from build123d import *

# Parameters (mm, degrees)
BOSS_EXTRUDE1_DEPTH = 3
SKETCH2_R           = 1.5
SKETCH2_W           = 57.5
SKETCH2_H           = 86
CUT_EXTRUDE1_DEPTH  = 102.651364969
SKETCH3_W           = 3
SKETCH3_H           = 15
CUT_EXTRUDE2_DEPTH  = 102.651364969


with BuildPart() as part:
    # Sketch1 → Boss-Extrude1 (new body)
    with BuildSketch(Plane(origin=(0, 0, 0), x_dir=(1, 0, 0), z_dir=(0, 1, 0))):
        with BuildLine():
            Line((-74, 60), (74, 60))
            ThreePointArc((74, 60), (79.656854249, 57.656854249), (82, 52))
            Line((82, 52), (82, -52))
            ThreePointArc((82, -52), (79.656854249, -57.656854249), (74, -60))
            Line((74, -60), (-74, -60))
            ThreePointArc((-74, -60), (-79.656854249, -57.656854249), (-82, -52))
            Line((-82, -52), (-82, 52))
            ThreePointArc((-82, 52), (-79.656854249, 57.656854249), (-74, 60))
        make_face()
    extrude(amount=BOSS_EXTRUDE1_DEPTH)

    # Sketch2 → Cut-Extrude1 (cut, through all)
    with BuildSketch(Plane(origin=(0, 3, 0), x_dir=(1, 0, 0), z_dir=(0, 1, 0))):
        with Locations(Location((-38.25, 50, 0), (0, 0, 270))):
            Circle(SKETCH2_R)
        with Locations(Location((-38.25, -50, 0), (0, 0, 270))):
            Circle(SKETCH2_R)
        with Locations((-38.25, -1.5)):
            Rectangle(SKETCH2_W, SKETCH2_H)
    extrude(amount=-CUT_EXTRUDE1_DEPTH, mode=Mode.SUBTRACT)

    # Sketch3 → Cut-Extrude2 (cut, through all)
    with BuildSketch(Plane(origin=(0, 3, 0), x_dir=(1, 0, 0), z_dir=(0, 1, 0))):
        with Locations((-72.5, 32.5)):
            Rectangle(SKETCH3_W, SKETCH3_H)
        with Locations((-72.5, -32.5)):
            Rectangle(SKETCH3_W, SKETCH3_H)
        with Locations((72.5, -32.5)):
            Rectangle(SKETCH3_W, SKETCH3_H)
        with Locations((72.5, 32.5)):
            Rectangle(SKETCH3_W, SKETCH3_H)
    extrude(amount=-CUT_EXTRUDE2_DEPTH, mode=Mode.SUBTRACT)


solid = part.part
Verification items for the finished model (mm, model axes). Round coordinates to 2 decimals unless told otherwise and drop trailing zeros. Loops run counter-clockwise (first coordinate to the right, second up) from the corner with the lowest first, then second, coordinate; pieces in that order, holes last. Notation, with made-up numbers: (-15.5, 56.5) - (34.5, 56.5) arc R26 ccw to (34.5, 81.5) - close; hole circle Ø1 at (65, -7). An arc over 180 degrees is marked (long way). Use a Markdown table: item, result. Add a question column.
1. Section check B-B, the plane z = -31. Record the boundary of the cut face in (x, y), plus the area to 4 significant figures.
2. Thickness scan on probe 1 along X at (y, z) = (0.6, 30.5); probe 2 along X at (y, z) = (1.35, 4); probe 3 along Z at (x, y) = (-13, 1.1). Record the ranges inside material, lowest first. Write a range as [from, to].
3. Gauge pin test, flat end, axial feed: pin 1 (2.5 mm diameter, centred on x = -38.25, z = -50, fed in from +Y). Record the tip position at first contact, or that the pin passes through.
4. Section check A-A, the plane z = -7. Record the boundary of the cut face in (x, y).
5. Section check D-D, the plane y = 2.55. Give the number of separate pieces and of enclosed holes in the cut face, plus the area to 3 significant figures.
6. Section check C-C, the plane x = -17. Record the boundary of the cut face in (y, z), plus the area to 3 significant figures.
Checks:
| question | item | result |
|---|---|---|
| 1 | outline | (-82, 0) - (-74, 0) - (-74, 3) - (-82, 3) - close; (-71, 0) - (-67, 0) - (-67, 3) - (-71, 3) - close; (-9.5, 0) - (71, 0) - (71, 3) - (-9.5, 3) - close; (74, 0) - (82, 0) - (82, 3) - (74, 3) - close |
| 1 | area | 301.5 mm^2 |
| 2 | probe 1 | x = [-82, -74], [-71, -67], [-9.5, 71], [74, 82] |
| 2 | probe 2 | x = [-82, -67], [-9.5, 82] |
| 2 | probe 3 | z = [-60, -41.5], [44.5, 60] |
| 3 | pin 1 | passes through |
| 4 | outline | (-82, 0) - (-67, 0) - (-67, 3) - (-82, 3) - close; (-9.5, 0) - (82, 0) - (82, 3) - (-9.5, 3) - close |
| 5 | separate pieces | 1 |
| 5 | enclosed holes | 7 |
| 5 | area | 14,500 mm^2 |
| 6 | outline | (0, -60) - (3, -60) - (3, -41.5) - (0, -41.5) - close; (0, 44.5) - (3, 44.5) - (3, 60) - (0, 60) - close |
| 6 | area | 102 mm^2 |
